from build123d import *

# Parameters (mm, degrees)
SKETCH1_W           = 13
SKETCH1_H           = 18
BOSS_EXTRUDE1_DEPTH = 3.4
SKETCH2_W           = 15
SKETCH2_H           = 20
BOSS_EXTRUDE2_DEPTH = 1
SKETCH4_R           = 1.5
CUT_EXTRUDE2_DEPTH  = 14.251792332
FILLET1_R           = 1


with BuildPart() as part:
    # Sketch1 → Boss-Extrude1 (new body)
    with BuildSketch(Plane(origin=(0, 0, 0), x_dir=(1, 0, 0), z_dir=(0, 1, 0))):
        Rectangle(SKETCH1_W, SKETCH1_H)
    extrude(amount=BOSS_EXTRUDE1_DEPTH)

    # Sketch2 → Boss-Extrude2 (add)
    with BuildSketch(Plane(origin=(0, 3.4, 0), x_dir=(1, 0, 0), z_dir=(0, 1, 0))):
        Rectangle(SKETCH2_W, SKETCH2_H)
    extrude(amount=BOSS_EXTRUDE2_DEPTH)

    # Sketch4 → Cut-Extrude2 (cut, through all)
    with BuildSketch(Plane.XZ):
        with BuildLine():
            Line((-2.5, 5.5), (-3.734023309, 6.734023309))
            ThreePointArc((-3.734023309, 6.734023309), (0, 7.7), (3.734023309, 6.734023309))
            Line((3.734023309, 6.734023309), (2.5, 5.5))
            Line((2.5, 5.5), (2.5, 2))
            ThreePointArc((2.5, 2), (2.629409523, 1.982962913), (2.75, 1.933012702))
            ThreePointArc((2.75, 1.933012702), (4.25, 1.933012702), (5, 3.232050808))
            ThreePointArc((5, 3.232050808), (5.146446609, 3.585604198), (5.5, 3.732050808))
            Line((5.5, 3.732050808), (5.5, 5.809475019))
            ThreePointArc((5.5, 5.809475019), (0, 8), (-5.5, 5.809475019))
            Line((-5.5, 5.809475019), (-5.5, 2.767949192))
            ThreePointArc((-5.5, 2.767949192), (-4.137600278, 3.685275378), (-2.5, 3.55923704))
            Line((-2.5, 3.55923704), (-2.5, 5.5))
        make_face()
        with Locations(Location((0, 3, 0), (0, 0, 270))):
            Circle(SKETCH4_R)
        with BuildLine():
            Line((-2.5, -0.94076296), (-2.5, 2.5))
            ThreePointArc((-2.5, 2.5), (-2.629409523, 2.517037087), (-2.75, 2.566987298))
            ThreePointArc((-2.75, 2.566987298), (-4.25, 2.566987298), (-5, 1.267949192))
            ThreePointArc((-5, 1.267949192), (-5.146446609, 0.914395802), (-5.5, 0.767949192))
            Line((-5.5, 0.767949192), (-5.5, -1.732050808))
            ThreePointArc((-5.5, -1.732050808), (-4.137600278, -0.814724622), (-2.5, -0.94076296))
        make_face()
        with BuildLine():
            ThreePointArc((5.5, 1.732050808), (4.137600278, 0.814724622), (2.5, 0.94076296))
            Line((2.5, 0.94076296), (2.5, -2.5))
            ThreePointArc((2.5, -2.5), (2.629409523, -2.517037087), (2.75, -2.566987298))
            ThreePointArc((2.75, -2.566987298), (4.25, -2.566987298), (5, -1.267949192))
            ThreePointArc((5, -1.267949192), (5.146446609, -0.914395802), (5.5, -0.767949192))
            Line((5.5, -0.767949192), (5.5, 1.732050808))
        make_face()
        with Locations(Location((0, -3, 0), (0, 0, 270))):
            Circle(SKETCH4_R)
        with BuildLine():
            Line((-2.5, -3), (-2.5, -2))
            ThreePointArc((-2.5, -2), (-2.629409523, -1.982962913), (-2.75, -1.933012702))
            ThreePointArc((-2.75, -1.933012702), (-4.25, -1.933012702), (-5, -3.232050808))
            ThreePointArc((-5, -3.232050808), (-5.146446609, -3.585604198), (-5.5, -3.732050808))
            Line((-5.5, -3.732050808), (-5.5, -8))
            Line((-5.5, -8), (0.192885679, -8))
            ThreePointArc((0.192885679, -8), (-0.966559904, -6.870975799), (-1.497403196, -5.342180487))
            ThreePointArc((-1.497403196, -5.342180487), (-1.489544615, -5.189572213), (-1.435960525, -5.046464603))
            ThreePointArc((-1.435960525, -5.046464603), (-2.218096178, -4.153277653), (-2.5, -3))
        make_face()
        with BuildLine():
            ThreePointArc((5.5, -2.767949192), (4.107029075, -3.693132835), (2.442465304, -3.533257199))
            ThreePointArc((2.442465304, -3.533257199), (1.376562779, -5.086881625), (-0.471204729, -5.455191663))
            ThreePointArc((-0.471204729, -5.455191663), (0.396247062, -6.922515496), (2, -7.5))
            ThreePointArc((2, -7.5), (2.353553391, -7.646446609), (2.5, -8))
            Line((2.5, -8), (5.5, -8))
            Line((5.5, -8), (5.5, -2.767949192))
        make_face()
    extrude(amount=-CUT_EXTRUDE2_DEPTH, mode=Mode.SUBTRACT)

    # Fillet1
    fillet1_edges = [part.edges().sort_by_distance(p)[0] for p in [
        (6.5, 1.7, 9),
        (-6.5, 1.7, 9),
        (-6.5, 1.7, -9),
        (6.5, 1.7, -9),
    ]]
    fillet(fillet1_edges, radius=FILLET1_R)


solid = part.part
Input: part model. Units: mm. Frame: model coordinates. A direction names the side the tool comes from. Round coordinates to 2 decimals unless told otherwise and drop trailing zeros. Loops run counter-clockwise (first coordinate to the right, second up) from the corner with the lowest first, then second, coordinate; pieces in that order, holes last. Notation, with made-up numbers: M -24.75,11 L 2.25,11 A28 cw 2.25,31 Z; hole C 30,22 d1. An arc over 180 degrees is marked long. Answer as CSV lines item,"result". Start each with the question number.
(1) Section C-C, the plane z = 3. Output: boundary loops of the cut face in (x, y), plus the area to 3 significant figures.
(2) Reachability of faces 4 (the flat face through (5.5, 2, 0)), 5 (the cylindrical face through (6.215, 1.724, -8.699)), 6 (the flat face through (-7.5, 4, 0)) from +Z, -Z, +X, -X, +Y, -Y: full face, straight path, thin tool, end or side. Return the list, or none.
(3) Draft query along X for faces 1 (the cylindrical face through (-6.199, 1.724, 8.715)), 2 (the cylindrical face through (4.23, 2.17, 1.92)), 3 (the flat face through (0, 4.4, 0)). Return one class per face: released by +X, released by -X, zero draft, split by the parting line, or undercut.
(4) First-contact query: pin 1 (2 mm diameter, centred on y = 1.5, z = -6, fed in from -X); pin 2 (2 mm diameter, centred on y = 2, z = 6, fed in from +X); pin 3 (1 mm diameter, centred on x = 2.5, y = 2, fed in from -Z). Flat tips, straight axial feed; report the tip coordinate or a pass-through.
(5) Section A-A, the plane z = 0.5. Output: boundary loops of the cut face in (x, y).
(6) Section D-D, the plane y = 4.1. State how many separate pieces and enclosed holes the cut face has, plus the area to 3 significant figures.
(7) Section B-B, the plane x = -2.25. Output: boundary loops of the cut face in (y, z), plus the area to 3 significant figures.
(8) Line query: line 1 (X direction, y = 3.75, z = 5); line 2 (X direction, y = 0.25, z = 0.5); line 3 (X direction, y = 3.45, z = 3). Output: solid intervals per line, ascending. Write a range as [from, to].
Values found:
1,outline,"M -7.5,3.4 L -6.5,3.4 L -6.5,0 L -5.5,0 L -5.5,4.4 L -7.5,4.4 Z; M -5.3,0 L -1.5,0 L -1.5,4.4 L -5.3,4.4 Z; M 1.5,0 L 2.5,0 L 2.5,4.4 L 1.5,4.4 Z; M 4.98,0 L 6.5,0 L 6.5,3.4 L 7.5,3.4 L 7.5,4.4 L 4.98,4.4 Z"
1,area,"34.2 mm²"
2,face 4,"+Y, -Y"
2,face 5,"-Z, +X, -Y"
2,face 6,"+Z, -Z, -X, +Y, -Y"
3,face 1,"released by -X"
3,face 2,"undercut"
3,face 3,"zero draft"
4,pin 1,"stops at x = -6.5"
4,pin 2,"stops at x = 6.5"
4,pin 3,"stops at z = -9"
5,outline,"M -7.5,3.4 L -6.5,3.4 L -6.5,0 L -5.5,0 L -5.5,4.4 L -7.5,4.4 Z; M -2.5,0 L 2.5,0 L 2.5,4.4 L -2.5,4.4 Z; M 5.5,0 L 6.5,0 L 6.5,3.4 L 7.5,3.4 L 7.5,4.4 L 5.5,4.4 Z"
6,separate pieces,"1"
6,enclosed holes,"7"
6,area,"202 mm²"
7,outline,"M 0,-9 L 3.4,-9 L 3.4,-10 L 4.4,-10 L 4.4,-8 L 0,-8 Z; M 0,-4.09 L 4.4,-4.09 L 4.4,7.36 L 0,7.36 Z; M 0,7.68 L 4.4,7.68 L 4.4,10 L 3.4,10 L 3.4,9 L 0,9 Z"
7,area,"62.6 mm²"
8,line 1,"x = [-7.5, -5.5], [-2.5, 2.5], [5.5, 7.5]"
8,line 2,"x = [-6.5, -5.5], [-2.5, 2.5], [5.5, 6.5]"
8,line 3,"x = [-7.5, -5.5], [-5.3, -1.5], [1.5, 2.5], [4.98, 7.5]"
